from build123d import *

# Parameters (mm, degrees)
F0_W        = 12.7
F0_H        = 94.5614505536
F1_DEPTH    = 2.54
F3_DEPTH    = 3.81
F4_R        = 1.905
F5_T1_DEPTH = 19.7995158286
F5_T3_DEPTH = 80.155505846


# Not quite as in the source:
# - a fillet or chamfer that OpenCascade refuses, or shapes differently, is made with other operations: its cross-section is extruded or revolved along the edge and cut away or added


with BuildPart() as f1:
    # F0 (on Top) → F1 (new body)
    with BuildSketch(Plane.XY):
        with Locations((-6.35, -5.6614459495)):
            Rectangle(F0_W, F0_H)
    extrude(amount=F1_DEPTH)

    # F2 (on face) → F3 (cut)
    with BuildSketch(Plane.XY.offset(2.54)):
        Polygon((-12.7, 17.6289882511), (-6.35, 41.6192793273), (-12.7, 41.6192793273), align=None)
        Polygon((0, 41.6192793273), (-6.35, 41.6192793273), (0, 17.6289882511), align=None)
    extrude(amount=-F3_DEPTH, mode=Mode.SUBTRACT)

    # F4
    f4_edges = [f1.edges().sort_by_distance(p)[0] for p in [
        (-3.175, 29.624134, 2.54),
        (-12.7, -17.656591, 2.54),
        (0, -17.656591, 2.54),
        (-6.35, -52.942171, 2.54),
        (-9.525, 29.624134, 2.54),
    ]]
    fillet(f4_edges, radius=F4_R)

    # F5: fillet of radius 1.905 on 3 edges, made by hand

    # F5_s2 → F5_t1 (cut)
    with BuildSketch(Plane.YZ.offset(-16.2497579143)):
        with BuildLine():
            ThreePointArc((-51.5222680606, 0), (-52.299981054, 0.1659808799), (-52.9421712264, 0.635))
            Line((-52.9421712264, 0.635), (-52.9421712264, 0))
            Line((-52.9421712264, 0), (-51.5222680606, 0))
        make_face()
    extrude(amount=F5_T1_DEPTH, mode=Mode.SUBTRACT)

    # F5_s4 → F5_t3 (cut)
    with BuildSketch(Plane.XZ.offset(-23.6635767054)):
        with BuildLine():
            ThreePointArc((-11.2800968343, 0), (-12.0578098276, 0.1659808799), (-12.7, 0.635))
            Line((-12.7, 0.635), (-12.7, 0))
            Line((-12.7, 0), (-11.2800968343, 0))
        make_face()
        with BuildLine():
            ThreePointArc((-1.4199031657, 0), (-0.6421901724, 0.1659808799), (0, 0.635))
            Line((0, 0.635), (0, 0))
            Line((0, 0), (-1.4199031657, 0))
        make_face()
    extrude(amount=F5_T3_DEPTH, mode=Mode.SUBTRACT)


solid = f1.part
Verification items for the finished model (mm, model axes). Round coordinates to 2 decimals unless told otherwise and drop trailing zeros. Order: outer loops, then holes, each group sorted by start corner. A loop starts at its lowest first (then second) coordinate and runs counter-clockwise, first axis right, second up.
1. Go/stop test with a flat-tipped pin: P1, Ø1, axis at x = -1.5, z = 2, coming from the -Y side. Record where the tip stops, or that it passes through.
Final values:
P1: stops at y = -52.73
2. Thickness scan on L1, parallel to X at y = -1, z = 0.75; L2, parallel to X at y = 21, z = 1.8; L3, parallel to Z at x = -11.5, y = 12. Record the ranges inside material, lowest first.
Final values:
L1: x = -12.7 to 0
L2: x = -11.4 to -1.3
L3: z = 0.01 to 2.4
3. Section check B-B on z = 1.25. Record the cut outline in (x, y).
Final values:
outline: (-12.6, -52.84) - (-0.1, -52.84) - (-0.1, 17.62) - (-6.35, 41.22) - (-12.6, 17.62) - close
4. Section check A-A on y = -33.5. Record the cut outline in (x, z) (3 decimals).
Final values:
outline: (-12.7, 0.635) arc R1.905 ccw to (-11.28, 0) - (-1.42, 0) arc R1.905 ccw to (0, 0.635) arc R1.905 ccw to (-1.905, 2.54) - (-10.795, 2.54) arc R1.905 ccw to start
